The figure shows three views and two pictorial views of one solid part (mm, origin at its lowest corner). Answer the questions. Coordinates: 2 decimals unless noted, no trailing zeros. Order: outer loops, then holes, each group sorted by start corner. A loop starts at its lowest first (then second) coordinate and runs counter-clockwise, first axis right, second up. Notation, with made-up numbers: (72.5, -9) -> (100.5, -9) arc R17 cw to (100.5, 2) -> close; hole circle Ø1 at (64, 14.25). An arc over 180 degrees is marked (long way). Write item = value, one per line. Start each with the question number.
Q1. The part is cut by section A-A, the plane x = 6. Determine the outline of the cut face in (y, z) (3 decimals).
Q2. A flat-ended cylindrical pin translates along its axis: pin 1 (2.5 mm diameter, centred on x = 6, y = 3.175, fed in from -Z). Find the tip coordinate at first contact, or state that the pin passes through.
Q3. Straight lines are drawn through the part: L1, parallel to Y at x = 6, z = 2.6 (3 decimals); L2, parallel to Y at x = 7.5, z = 3.5; L3, parallel to Y at x = 44, z = 1.55. For each, find the intervals that lie inside material, in ascending order. Write a range as from..to.
Q4. For a pull along X with two mould halves and no side action, classify the marked faces 1, 2 and 3 as +X half, -X half, draft (parallel to the pull), parting line (faces both ways), or undercut.
Q5. The part is cut by section C-C, the plane z = 2.1. Determine the outline of the cut face in (x, y) (3 decimals), plus the area to 3 significant figures.
Q6. The part is cut by section B-B, the plane y = 2.5. Determine the outline of the cut face in (x, z), plus the area to 3 significant figures.
Q7. The part is cut by section D-D, the plane x = 20.5. Determine the outline of the cut face in (y, z), plus the area to 3 significant figures.
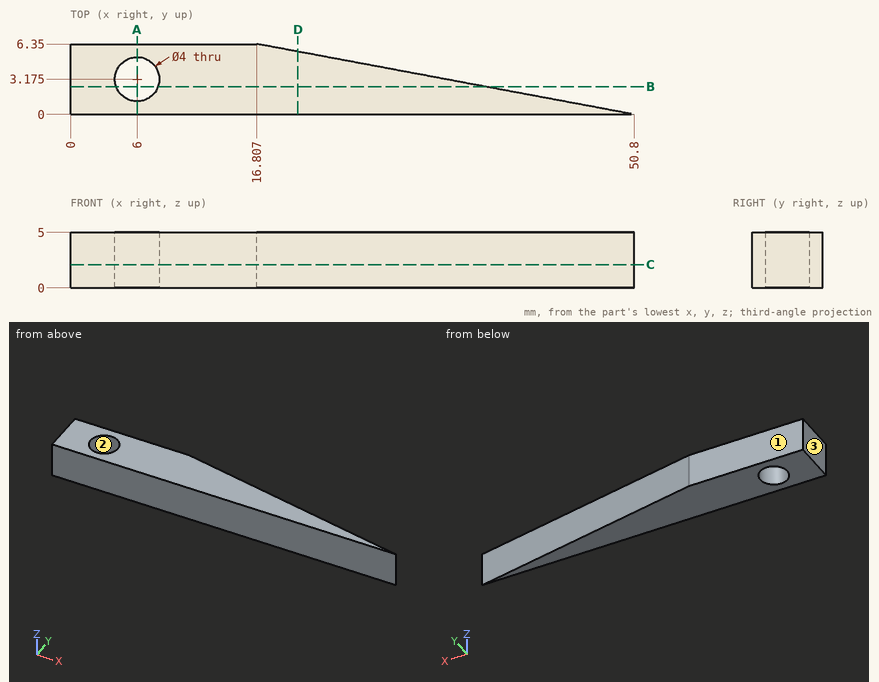
Model answer:
q1.outline = (0, 0) -> (1.175, 0) -> (1.175, 5) -> (0, 5) -> close; (5.175, 0) -> (6.35, 0) -> (6.35, 5) -> (5.175, 5) -> close
q2.pin_1 = through
q3.L1 = 0..1.175, 5.175..6.35
q3.L2 = 0..1.85, 4.5..6.35
q3.L3 = 0..1.27
q4.face_1 = draft
q4.face_2 = undercut
q4.face_3 = -X half
q5.outline = (0, 0) -> (50.8, 0) -> (16.807, 6.35) -> (0, 6.35) -> close; hole circle Ø4 at (6, 3.175)
q5.area = 202 mm2
q6.outline = (0, 0) -> (4.12, 0) -> (4.12, 5) -> (0, 5) -> close; (7.88, 0) -> (37.42, 0) -> (37.42, 5) -> (7.88, 5) -> close
q6.area = 168 mm2
q7.outline = (0, 0) -> (5.66, 0) -> (5.66, 5) -> (0, 5) -> close
q7.area = 28.3 mm2
